Model file for the job. Use its own axes, mm. A direction names the side the tool comes from. Give positions to 0.01 mm unless a question says otherwise; leave off trailing zeros. Write each loop counter-clockwise with the first axis right and the second up, starting at its lowest first coordinate (ties: lowest second). Pieces come first, ordered by that corner, then holes. Notation, with made-up numbers: M 65,-39 L 101,-39 A35 cw 101,-4 Z; hole C 6,9 d5. An arc over 180 degrees is marked long. Answer as a JSON object with one key per item and string values. Group by question number.
Autodesk Inventor part; units mm, degrees
ref_plane "YZ Plane" through (0, 0, 0) normal (1, 0, 0) x (0, 1, 0)
ref_plane "XZ Plane" through (0, 0, 0) normal (0, 1, 0) x (-1, 0, 0)
ref_plane "XY Plane" through (0, 0, 0) normal (0, 0, 1) x (1, 0, 0)
sketch "Sketch1" plane through (0, 0, 0) normal (0, 0, 1) x (1, 0, 0)
  point P0 (0, 0)
sketch "Sketch2" plane through (0, 0, 0) normal (0, 0, 1) x (1, 0, 0)
  circle A0 centre (0, 0) radius 73.505
  circle A1 centre (0, 0) radius 84.555
  line L0 (0, 0) -> (0, 267.2238)
  line L1 (0, 73.505) -> (0, 78.2675)
  circle A2 centre (0, 78.2675) radius 4.7625
  circle A3 centre (-46.0045, 63.3197) radius 4.7625
  circle A4 centre (-74.4368, 24.186) radius 4.7625
  circle A5 centre (-74.4368, -24.186) radius 4.7625
  circle A6 centre (-46.0045, -63.3197) radius 4.7625
  circle A7 centre (0, -78.2675) radius 4.7625
  circle A8 centre (46.0045, -63.3197) radius 4.7625
  circle A9 centre (74.4368, -24.186) radius 4.7625
  circle A10 centre (74.4368, 24.186) radius 4.7625
  circle A11 centre (46.0045, 63.3197) radius 4.7625
  point P0 (0, 73.505)
  point P1 (43.2052, 59.4668)
  point P2 (69.9074, 22.7143)
  point P3 (69.9074, -22.7143)
  point P4 (43.2052, -59.4668)
  point P5 (0, -73.505)
  point P6 (-43.2052, -59.4668)
  point P7 (-69.9074, -22.7143)
  point P8 (-69.9074, 22.7143)
  point P9 (-43.2052, 59.4668)
  dimension "d0" = 147.01
  dimension "d1" = 169.11
  dimension "d3" = 4.7625
  dimension "d4" = 9.525
  dimension "d7" = 360
extrude "Extrusion1" add sketch "Sketch2" along normal blind 3
sketch "Sketch3" plane through (0, 0, 3) normal (0, 0, 1) x (1, 0, 0)
  circle A0 centre (0, 0) radius 84.555
  line L0 (0, 84.555) -> (0, 84.055)
  line L1 (0.25, 83.8031) -> (-0.25, 83.8031)
  line L2 (-0.25, 83.8031) -> (-0.25, 84.3031)
  line L3 (-0.25, 84.3031) -> (0.25, 84.3031)
  line L4 (0.25, 84.3031) -> (0.25, 83.8031)
  line L5 (0.25, 83.8031) -> (-0.25, 84.3031) construction
  line L6 (-0.25, 83.8031) -> (0.25, 84.3031) construction
  point P0 (0, 84.0531)
  dimension "d11" = 0.5
  dimension "d15" = 0.5
  dimension "d16" = 0.5
extrude "Extrusion2" cut sketch "Sketch3" against normal blind 10 contours L1 L2 L3 L4
properties part number "bracket 1" material "Stainless Steel"
Q1. Wall check: L1, parallel to Y at x = 44.5, z = 1.9; L2, parallel to X at y = 66, z = 2.8; L3, parallel to Y at x = -50, z = 1.65. Give the ranges that are in metal, low to high.
Q2. Two-plate mould, pull along X, no slides. Class faces 3 (the cylindrical face through (80.65, -25.4, 1.48)), 4 (the flat face through (-25.4, 69.3, 0)), 5 (the cylindrical face through (-22.407, -70.007, 1.479)), 6 (the cylindrical face through (-23.022, 69.807, 1.479)): +X half, -X half, draft (parallel to the pull), parting line (faces both ways), or undercut.
Q3. Slice it at A-A, the plane y = 0. Write the cut outline in (x, z) (3 decimals), then the cut area to 3 significant figures.
Q4. Slice it at B-B, the plane x = -17. Write the cut outline in (y, z).
Q5. 3-axis set-ups, long thin cutter, end or side, ignore diameter. For faces 1 (the flat face through (-25.4, 69.3, 3)), 2 (the cylindrical face through (59.276, 43.466, 1.479)): which of +Z, -Z, +X, -X, +Y, -Y reach the whole face in a straight line?
Solved:
{
 "1": {"L1": "y = -71.9 to -67.84, -58.8 to -58.5, 58.5 to 58.8, 67.84 to 71.9", "L2": "x = -52.85 to -49.94, -42.07 to -32.36, 32.36 to 42.07, 49.94 to 52.85", "L3": "y = -68.19 to -65.91, -60.73 to -53.88, 53.88 to 60.73, 65.91 to 68.19"},
 "2": {"face 3": "parting line", "face 4": "draft", "face 5": "undercut", "face 6": "undercut"},
 "3": {"outline": "M -84.555,0 L -73.505,0 L -73.505,3 L -84.555,3 Z; M 73.505,0 L 84.555,0 L 84.555,3 L 73.505,3 Z", "area": "66.3 mm²"},
 "4": {"outline": "M -82.83,0 L -71.51,0 L -71.51,3 L -82.83,3 Z; M 71.51,0 L 82.83,0 L 82.83,3 L 71.51,3 Z"},
 "5": {"face 1": "+Z, +X, -X, +Y, -Y", "face 2": "+Z, -Z"}
}
